Autodesk Inventor part; units mm, degrees
ref_plane "YZ Plane" through (0, 0, 0) normal (1, 0, 0) x (0, 1, 0)
ref_plane "XZ Plane" through (0, 0, 0) normal (0, 1, 0) x (-1, 0, 0)
ref_plane "XY Plane" through (0, 0, 0) normal (0, 0, 1) x (1, 0, 0)
sketch "Sketch1" plane through (0, 0, 0) normal (0, 1, 0) x (-1, 0, 0)
  line L0 (0, 0) -> (0, -150)
  line L1 (0, -150) -> (50, -150)
  line L2 (0, 0) -> (50, -44.9152) construction
  line L3 (50, -44.9152) -> (50, -150) construction
  spline S0 degree 2 poles (0, 0) (50, -44.9152) (50, -150) knots 1 1 1 2 2 2
  dimension "d0" = 150
  dimension "d2" = 50
revolve "Revolution1" add sketch "Sketch1" angle 90 about axis through (0, 0, -150) along (-1, 0, 0)
sketch "Sketch2" plane through (0, 0, -150) normal (0, 0, -1) x (-1, 0, 0)
  line L0 (0, 150) -> (0, 0)
  line L1 (0, 0) -> (50, 0)
  line L2 (0, 0) -> (20, 0)
  line L3 (20, 0) -> (20, 50)
  line L4 (15, 55) -> (25, 55)
  line L5 (25, 55) -> (25, 45)
  line L6 (25, 45) -> (15, 45)
  line L7 (15, 45) -> (15, 55)
  line L8 (15, 55) -> (25, 45) construction
  line L9 (25, 55) -> (15, 45) construction
  dimension "d9" = 20
  dimension "d10" = 50
  dimension "d11" = 10
  dimension "d12" = 10
extrude "Extrusion1" add sketch "Sketch2" along normal blind 10
sketch "Sketch3" plane through (-50, 0, -150) normal (0, -1, 0) x (1, 0, 0)
  line L0 (50, 0) -> (30, 0)
  line L1 (50, 0) -> (0, 0)
  line L2 (30, 0) -> (30, 50)
  line L3 (35.1, 44.9) -> (24.9, 44.9)
  line L4 (24.9, 44.9) -> (24.9, 55.1)
  line L5 (24.9, 55.1) -> (35.1, 55.1)
  line L6 (35.1, 55.1) -> (35.1, 44.9)
  line L7 (35.1, 44.9) -> (24.9, 55.1) construction
  line L8 (24.9, 44.9) -> (35.1, 55.1) construction
  point P0 (50, 150)
  dimension "d19" = 20
  dimension "d20" = 50
  dimension "d21" = 10.2
  dimension "d22" = 10.2
extrude "Extrusion2" cut sketch "Sketch3" against normal blind 10
sketch "Sketch4" plane through (0, 0, 0) normal (1, 0, 0) x (0, 0, -1)
  line L0 (0, 0) -> (150, 0)
  line L1 (150, 0) -> (150, 75)
  line L2 (150, 150) -> (150, 0)
  line L3 (150, 75) -> (75, 75)
  circle A0 centre (75, 75) radius 6.25
  line L4 (75, 75) -> (75, 64)
  line L5 (75, 75) -> (84.5263, 69.5)
  line L6 (75, 75) -> (84.5263, 80.5)
  line L7 (75, 75) -> (75, 86)
  line L8 (75, 75) -> (65.4737, 80.5)
  line L9 (75, 75) -> (65.4737, 69.5)
  line L10 (75, 64) -> (65.4737, 69.5)
  line L11 (65.4737, 69.5) -> (65.4737, 80.5)
  line L12 (65.4737, 80.5) -> (75, 86)
  line L13 (75, 86) -> (84.5263, 80.5)
  line L14 (84.5263, 80.5) -> (84.5263, 69.5)
  line L15 (84.5263, 69.5) -> (75, 64)
  dimension "d25" = 75
  dimension "d26" = 75
  dimension "d27" = 12.5
  dimension "d33" = 11
  dimension "d36" = 360
extrude "Extrusion5" cut sketch "Sketch4" against normal blind 59.85
extrude "Extrusion6" add sketch "Sketch4" against normal blind 5 contours A0 L6 L14 L3 | L3 L14 L5 A0 | A0 L7 L13 L6 | L5 L15 L4 A0 | L4 L10 L9 A0 | A0 L8 L12 L7 | A0 L9 L11 L8
properties part number "3DPrintShapeCorner"
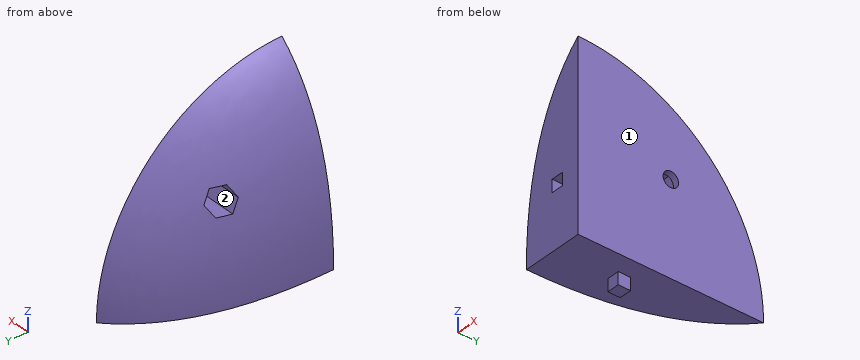
Work out the finished part from the listing and answer in its coordinate system (mm). Face numbers are marked on the shaded views. Give positions to 0.01 mm unless a question says otherwise; leave off trailing zeros. Put each result on its own line as item: value. Start each with the question number.
Item 1: Find the intervals of material crossed by L1, parallel to Y at x = -3.85, z = -75; L2, parallel to Y at x = -3.05, z = -75; L3, parallel to Z at x = -3, y = 75, in increasing order. Write a range as [from, to].
Item 2: Each of these flat-tipped pins is pushed along its axis until it touches: P1, Ø12, axis at x = -14, y = 74, coming from the -Z side; P2, Ø15, axis at x = -14, y = 55.5, coming from the -Z side; P3, Ø9.5, axis at y = 70, z = -76.5, coming from the -X side; P4, Ø5, axis at x = -18.5, z = -154, coming from the -Y side. Where does it stop, or does it pass through?
Item 3: The mould has two halves that part along Z. Classify the marked faces 1 and 2: released by +Z, released by -Z, zero draft, split by the parting line, or undercut.
Answers below:
1. L1: [0, 68.75], [81.25, 125.71]
1. L2: [0, 68.75], [81.25, 126.61]
1. L3: [-150, -81.25], [-68.75, -23.33]
2. P1: z = -150
2. P2: z = -160
2. P3: x = -35.12
2. P4: y = 45
3. face 1: zero draft
3. face 2: undercut
